Source: CAD feature listing. Evaluate the final solid. Frame: model axes, mm. Face numbers are marked on the shaded views. A direction names the side the tool comes from. Coordinates: 2 decimals unless noted, no trailing zeros. Loops run counter-clockwise (first coordinate to the right, second up) from the corner with the lowest first, then second, coordinate; pieces in that order, holes last. Notation, with made-up numbers: (-4, 15) -> (6, 15) arc R23 cw to (6, 39) -> close; hole circle Ø6 at (28.5, 43). An arc over 180 degrees is marked (long way). Answer as CSV lines item,"result".
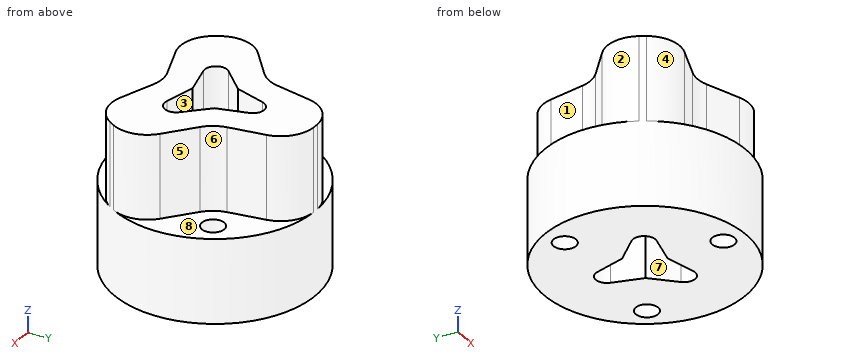
from build123d import *

# Parameters (mm, degrees)
SKETCH1_R                = 18
BOSS_EXTRUDE1_DEPTH      = 30
SKETCH2_R                = 2
CUT_EXTRUDE1_DEPTH       = 40
CUT_EXTRUDE2_DEPTH       = 15
FILLET2_R                = 6
CIRPATTERN3_COUNT        = 3
FILLET2_OF_CIRPATTERN3_R = 6
CUT_EXTRUDE3_START       = -30
CUT_EXTRUDE3_DEPTH       = 30
FILLET3_R                = 2


with BuildPart() as part:
    # Sketch1 → Boss-Extrude1 (new body)
    with BuildSketch(Plane.XY):
        Circle(SKETCH1_R)
    extrude(amount=BOSS_EXTRUDE1_DEPTH)

    # Sketch2 → Cut-Extrude1 (cut)
    with BuildSketch(Plane(origin=(0, 0, 0), x_dir=(-1, 0, 0), z_dir=(0, 0, -1))):
        with Locations((12.124355653, 7)):
            Circle(SKETCH2_R)
    cut_extrude1 = extrude(amount=-CUT_EXTRUDE1_DEPTH, mode=Mode.SUBTRACT)

    # Sketch3 → Cut-Extrude2 (cut)
    with BuildSketch(Plane.XY.offset(30)):
        Polygon((-15.686533479, 14.830127019), (-20.686533479, 6.169872981), (-17.60824379, -3.734936498), (-7.794228634, 4.5), (-5.569572007, 17.116654687), align=None)
    cut_extrude2 = extrude(amount=-CUT_EXTRUDE2_DEPTH, mode=Mode.SUBTRACT)

    # Fillet2
    fillet2_edges = [part.edges().sort_by_distance(p)[0] for p in [
        (-7.794228634, 4.5, 22.5),
        (-17.60824379, -3.734936498, 22.5),
        (-5.569572007, 17.116654687, 22.5),
    ]]
    fillet(fillet2_edges, radius=FILLET2_R)

    # CirPattern3: Cut-Extrude1, Cut-Extrude2 ×3 about axis
    cirpattern3_axis = Axis((0, 0, 0), (0, 0, 1))
    for i in range(1, CIRPATTERN3_COUNT):
        add(cut_extrude1.rotate(cirpattern3_axis, i * 360 / CIRPATTERN3_COUNT), mode=Mode.SUBTRACT)
        add(cut_extrude2.rotate(cirpattern3_axis, i * 360 / CIRPATTERN3_COUNT), mode=Mode.SUBTRACT)

    # Fillet2 of CirPattern3
    fillet2_of_cirpattern3_edges = [part.edges().sort_by_distance(p)[0] for p in [
        (0, -9, 22.5),
        (12.038671783, -13.381718189, 22.5),
        (-12.038671783, -13.381718189, 22.5),
        (7.794228634, 4.5, 22.5),
        (5.569572007, 17.116654687, 22.5),
        (17.60824379, -3.734936498, 22.5),
    ]]
    fillet(fillet2_of_cirpattern3_edges, radius=FILLET2_OF_CIRPATTERN3_R)

    # Sketch4 → Cut-Extrude3 (cut)
    with BuildSketch(Plane.XY.offset(30).offset(CUT_EXTRUDE3_START)):
        Polygon((-12.124355653, -7), (-3.464101615, 2), (0, 14), (3.464101615, 2), (12.124355653, -7), (0, -4), align=None)
    extrude(amount=CUT_EXTRUDE3_DEPTH, mode=Mode.SUBTRACT)

    # Fillet3
    fillet3_edges = [part.edges().sort_by_distance(p)[0] for p in [
        (12.124355653, -7, 15),
        (-12.124355653, -7, 15),
        (0, 14, 15),
    ]]
    fillet(fillet3_edges, radius=FILLET3_R)


solid = part.part
(1) Cut plane B-B (x = -13). Return the cut outline in (y, z), then the cut area to 3 significant figures.
Computed values:
outline,"(-12.45, 0) -> (5.2, 0) -> (5.2, 15) -> (0.13, 15) -> (0.13, 30) -> (-11.63, 30) -> (-11.63, 15) -> (-12.45, 15) -> close; (8.8, 0) -> (12.45, 0) -> (12.45, 15) -> (8.8, 15) -> close"
area,"496 mm^2"
(2) Material intervals for L1, parallel to Y at x = 0, z = 11; L2, parallel to Z at x = -4, y = -14; L3, parallel to X at y = -14, z = 10.5, sorted ascending. Write a range as [from, to].
Computed values:
L1,"[-18, -16], [-12, -4], [8.79, 18]"
L2,"[0, 15]"
L3,"[-11.31, -2], [2, 11.31]"
(3) Cut plane D-D (y = -7.5). Return the cut outline in (x, z), then the cut area to 3 significant figures.
Computed values:
outline,"(-16.36, 0) -> (16.36, 0) -> (16.36, 15) -> (16.29, 15) -> (16.29, 30) -> (-16.29, 30) -> (-16.29, 15) -> (-16.36, 15) -> close"
area,"980 mm^2"
(4) Cut plane C-C (z = 16.5). Return the cut outline in (x, y), then the cut area to 3 significant figures.
Computed values:
outline,"(-15.87, -8.5) arc R18 ccw to (-15.3, -9.49) arc R6 ccw to (-8.14, -11.96) -> (-2.05, -9.75) arc R6 cw to (2.05, -9.75) -> (8.14, -11.96) arc R6 ccw to (15.3, -9.49) arc R18 ccw to (15.87, -8.5) arc R6 ccw to (14.43, -1.07) -> (9.47, 3.1) arc R6 cw to (7.42, 6.65) -> (6.29, 13.04) arc R6 ccw to (0.57, 17.99) arc R18 ccw to (-0.57, 17.99) arc R6 ccw to (-6.29, 13.04) -> (-7.42, 6.65) arc R6 cw to (-9.47, 3.1) -> (-14.43, -1.07) arc R6 ccw to start; hole (-7.32, -2.01) arc R2 ccw to (-5.4, -5.34) -> (0, -4) -> (5.4, -5.34) arc R2 ccw to (7.32, -2.01) -> (3.46, 2) -> (1.92, 7.34) arc R2 ccw to (-1.92, 7.34) -> (-3.46, 2) -> close"
area,"492 mm^2"
(5) Cut plane A-A (y = 0). Return the cut outline in (x, z), then the cut area to 3 significant figures.
Computed values:
outline,"(-18, 0) -> (-5.39, 0) -> (-5.39, 30) -> (-13.16, 30) -> (-13.16, 15) -> (-18, 15) -> close; (5.39, 0) -> (18, 0) -> (18, 15) -> (13.16, 15) -> (13.16, 30) -> (5.39, 30) -> close"
area,"611 mm^2"
(6) Draft query along X for the marked faces 6, 7 and 8. Return one class per face: released by +X, released by -X, zero draft, split by the parting line, or undercut.
Computed values:
face 6,"released by +X"
face 7,"undercut"
face 8,"zero draft"
(7) Access query for the marked faces 1, 2, 3, 4 and 5. Directions: +Z, -Z, +X, -X, +Y, -Y. A direction counts if a zero-diameter tool reaches every point of the face in a straight line with its end or side. Return the directions, or none.
Computed values:
face 1,"+Z, -X, +Y"
face 2,"+Z, -X"
face 3,"+Z, -Z"
face 4,"+Z, -Y"
face 5,"+Z, +X, +Y"
(8) Pin query (flat end, axial travel): pin 1 Ø1 at (x, z) = (-6.5, 18.5) entering from -Y; pin 2 Ø2.5 at (x, y) = (2.5, -14) entering from +Z; pin 3 Ø10 at (y, z) = (6.5, 3.5) entering from -X. Return the tip coordinate at first contact, or that it passes through.
Computed values:
pin 1,"y = -11.55"
pin 2,"z = 15"
pin 3,"x = -17.94"
